Source: CAD feature listing. Evaluate the final solid. Frame: model axes, mm. A direction names the side the tool comes from. Round coordinates to 2 decimals unless told otherwise and drop trailing zeros. Loops run counter-clockwise (first coordinate to the right, second up) from the corner with the lowest first, then second, coordinate; pieces in that order, holes last. Notation, with made-up numbers: (-10.75, 52) - (21.25, 52) arc R23 cw to (21.25, 70) - close; hole circle Ø7 at (34.25, 36.25). An arc over 180 degrees is marked (long way). One line per question, with ' | ' between items.
from build123d import *

# Parameters (mm, degrees)
SKETCH1_R           = 1.5
BOSS_EXTRUDE1_DEPTH = 5
FILLET1_R           = 3
BOSS_EXTRUDE2_START = -5
BOSS_EXTRUDE2_DEPTH = 5


with BuildPart() as part:
    # Sketch1 → Boss-Extrude1 (new body)
    with BuildSketch(Plane.XY):
        with BuildLine():
            Line((-15.5, -3), (-12.5, -3))
            Line((-12.5, -3), (-4.5, -3))
            ThreePointArc((-4.5, -3), (-0.5, -5), (3.5, -3))
            ThreePointArc((3.5, -3), (4.5, 0), (3.5, 3))
            ThreePointArc((3.5, 3), (-0.5, 5), (-4.5, 3))
            Line((-4.5, 3), (-12.5, 3))
            Line((-12.5, 3), (-15.5, 3))
            Line((-15.5, 3), (-15.5, -3))
        make_face()
        with Locations((-0.5, 0)):
            Circle(SKETCH1_R, mode=Mode.SUBTRACT)
    extrude(amount=BOSS_EXTRUDE1_DEPTH)

    # Fillet1
    fillet1_edges = [part.edges().sort_by_distance(p)[0] for p in [
        (-15.5, -3, 2.5),
    ]]
    fillet(fillet1_edges, radius=FILLET1_R)

    # Sketch2 → Boss-Extrude2 (add)
    with BuildSketch(Plane.XY.offset(5).offset(BOSS_EXTRUDE2_START)):
        with BuildLine():
            Line((4.130629225, -1.886073429), (69.840963555, 7.16038973))
            ThreePointArc((69.840963555, 7.16038973), (71.97663963, 9.977992914), (69.159036445, 12.113668989))
            Line((69.159036445, 12.113668989), (3.448702116, 3.06720583))
            ThreePointArc((3.448702116, 3.06720583), (4.453279259, 0.681927109), (4.130629225, -1.886073429))
        make_face()
    extrude(amount=BOSS_EXTRUDE2_DEPTH)


solid = part.part
1. Section query B-B, the plane z = 2.75. Return loops of the section in (x, y), plus the area to 3 significant figures.
Worked out:
outline: (-15.5, 0) arc R3 ccw to (-12.5, -3) - (-4.5, -3) arc R5 ccw to (4.13, -1.89) - (69.84, 7.16) arc R2.5 ccw to (69.16, 12.11) - (3.45, 3.07) arc R5 ccw to (-4.5, 3) - (-15.5, 3) - close; hole circle Ø3 at (-0.5, 0) | area: 471 mm2
2. Contact query for flat-ended pins moving along their axis: P1, Ø1, axis at x = 43, z = 2, coming from the -Y side; P2, Ø2.5, axis at x = -10, z = 3.5, coming from the -Y side; P3, Ø1.5, axis at x = -9, z = 1.5, coming from the +Y side. Output: stop coordinate, or through.
Worked out:
P1: stops at y = 3.4 | P2: stops at y = -3 | P3: stops at y = 3
3. Material intervals for probe 1 along Y at (x, z) = (-0.5, 3.85); probe 2 along Y at (x, z) = (-11.5, 1.45); probe 3 along Y at (x, z) = (55, 4.6), sorted ascending.
Worked out:
probe 1: y = -5 to -1.5, 1.5 to 5 | probe 2: y = -3 to 3 | probe 3: y = 5.12 to 10.16
4. Section query C-C, the plane x = 53.5. Return loops of the section in (y, z).
Worked out:
outline: (4.91, 0) - (9.96, 0) - (9.96, 5) - (4.91, 5) - close
5. Section query D-D, the plane y = 8.25. Return loops of the section in (x, z).
Worked out:
outline: (41.09, 0) - (71.58, 0) - (71.58, 5) - (41.09, 5) - close
6. Section query A-A, the plane x = -0.5. Return loops of the section in (y, z), plus the area to 3 significant figures.
Worked out:
outline: (-5, 0) - (-1.5, 0) - (-1.5, 5) - (-5, 5) - close; (1.5, 0) - (5, 0) - (5, 5) - (1.5, 5) - close | area: 35.0 mm2
7. Mould query, pull axis X, two halves, no side actions, for faces 6 (the cylindrical face through (1, 0, 2)), 7 (the flat face through (-15.5, 2, 2)), 8 (the cylindrical face through (-0.5, 5, 2.5)), 9 (the flat face through (25, 4, 0)). Classes: released by +X, released by -X, zero draft, split by the parting line, or undercut.
Worked out:
face 6: undercut | face 7: released by -X | face 8: undercut | face 9: zero draft
8. Access query for faces 1 (the flat face through (-9, -3, 2)), 2 (the flat face through (36.526, 2.574, 2.465)), 3 (the flat face through (36.764, 7.654, 2.465)), 4 (the flat face through (25, 4, 5)), 5 (the flat face through (-10, 3, 2)). Directions: +Z, -Z, +X, -X, +Y, -Y. A direction counts if a zero-diameter tool reaches every point of the face in a straight line with its end or side. Return the directions, or none.
Worked out:
face 1: +Z, -Z, -X, -Y | face 2: +Z, -Z, +X, -Y | face 3: +Z, -Z, +Y | face 4: +Z, +X, -X, +Y, -Y | face 5: +Z, -Z, -X, +Y
